Build history of the part. All positions in model axes, mm. Face numbers are marked on the shaded views. Round coordinates to 2 decimals unless told otherwise and drop trailing zeros. Write each loop counter-clockwise with the first axis right and the second up, starting at its lowest first coordinate (ties: lowest second). Pieces come first, ordered by that corner, then holes. Notation, with made-up numbers: M 41.25,43.5 L 49.25,43.5 A25 cw 49.25,65.5 Z; hole C 83,79 d2. An arc over 180 degrees is marked long. Use a Markdown table: item, result.
from build123d import *

# Parameters (mm, degrees)
SKETCH1_W           = 76.2
SKETCH1_H           = 50.8
SKETCH1_R           = 14.2748
BOSS_EXTRUDE1_DEPTH = 3.175
SKETCH2_R           = 22.225
BOSS_EXTRUDE2_DEPTH = 4.445
SKETCH3_R           = 14.2748
CUT_EXTRUDE1_DEPTH  = 92.688810795
SKETCH4_R           = 15.8623
CUT_EXTRUDE2_DEPTH  = 1.6002
FILLET1_R           = 2.54
FILLET2_R           = 2.54
SKETCH5_R           = 2.54
CUT_EXTRUDE3_DEPTH  = 92.688810795


with BuildPart() as part:
    # Sketch1 → Boss-Extrude1 (new body)
    with BuildSketch(Plane(origin=(0, 0, 0), x_dir=(1, 0, 0), z_dir=(0, 1, 0))):
        with Locations((38.1, 25.4)):
            Rectangle(SKETCH1_W, SKETCH1_H)
        with Locations(Location((38.1, 25.4, 0), (0, 0, 270))):
            Circle(SKETCH1_R, mode=Mode.SUBTRACT)
    extrude(amount=BOSS_EXTRUDE1_DEPTH)

    # Sketch2 → Boss-Extrude2 (add)
    with BuildSketch(Plane(origin=(0, 3.175, 0), x_dir=(1, 0, 0), z_dir=(0, 1, 0))):
        with Locations(Location((38.1, 25.4, 0), (0, 0, 90))):
            Circle(SKETCH2_R)
    extrude(amount=BOSS_EXTRUDE2_DEPTH)

    # Sketch3 → Cut-Extrude1 (cut, through all)
    with BuildSketch(Plane.XZ.offset(-3.175)):
        with Locations(Location((38.1, -25.4, 0), (0, 0, 270))):
            Circle(SKETCH3_R)
    extrude(amount=-CUT_EXTRUDE1_DEPTH, mode=Mode.SUBTRACT)

    # Sketch4 → Cut-Extrude2 (cut)
    with BuildSketch(Plane(origin=(0, 0, 0), x_dir=(-1, 0, 0), z_dir=(0, -1, 0))):
        with Locations(Location((-38.332507849, 25.4, 0), (0, 0, 90))):
            Circle(SKETCH4_R)
    extrude(amount=-CUT_EXTRUDE2_DEPTH, mode=Mode.SUBTRACT)

    # Fillet1
    fillet1_edges = [part.edges().sort_by_distance(p)[0] for p in [
        (38.1, 3.175, -3.175),
    ]]
    fillet(fillet1_edges, radius=FILLET1_R)

    # Fillet2
    fillet2_edges = [part.edges().sort_by_distance(p)[0] for p in [
        (0, 1.5875, -50.8),
        (76.2, 1.5875, -50.8),
        (76.2, 1.5875, 0),
        (0, 1.5875, 0),
    ]]
    fillet(fillet2_edges, radius=FILLET2_R)

    # Sketch5 → Cut-Extrude3 (cut, through all)
    with BuildSketch(Plane(origin=(0, 3.175, 0), x_dir=(1, 0, 0), z_dir=(0, 1, 0))):
        with Locations(Location((69.85, 41.275, 0), (0, 0, 270))):
            Circle(SKETCH5_R)
        with Locations(Location((69.85, 9.525, 0), (0, 0, 270))):
            Circle(SKETCH5_R)
        with Locations(Location((6.35, 9.525, 0), (0, 0, 270))):
            Circle(SKETCH5_R)
        with Locations(Location((6.35, 41.275, 0), (0, 0, 270))):
            Circle(SKETCH5_R)
    extrude(amount=-CUT_EXTRUDE3_DEPTH, mode=Mode.SUBTRACT)


solid = part.part
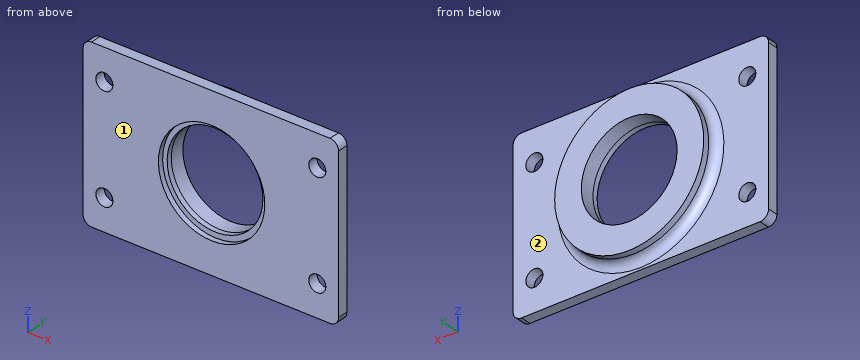
Q1. Drill centre lines: L1, parallel to X at y = 2.2, z = -25.4; L2, parallel to Y at x = 70, z = -20.5 (3 decimals); L3, parallel to Y at x = 27.5, z = -14. Where is each one in solid material? Low to high.
Response values:
| item | result |
|---|---|
| L1 | x = 0 to 23.83, 52.37 to 76.2 |
| L2 | y = 0 to 3.175 |
| L3 | y = 1.6 to 7.62 |
Q2. Cut at B-B on z = -25.4. Give the cut face in (x, y) (3 decimals), and give its area (3 significant figures).
Response values:
| item | result |
|---|---|
| outline | M 0,0 L 22.47,0 L 22.47,1.6 L 23.825,1.6 L 23.825,7.62 L 15.875,7.62 L 15.875,5.715 A2.54 cw 13.335,3.175 L 0,3.175 Z; M 52.375,1.6 L 54.195,1.6 L 54.195,0 L 76.2,0 L 76.2,3.175 L 62.865,3.175 A2.54 cw 60.325,5.715 L 60.325,7.62 L 52.375,7.62 Z |
| area | 220 mm2 |
Q3. Cut at A-A on x = 69.85. Give the cut face in (y, z) (3 decimals), and give its area (3 significant figures).
Response values:
| item | result |
|---|---|
| outline | M 0,-50.8 L 3.175,-50.8 L 3.175,-43.815 L 0,-43.815 Z; M 0,-38.735 L 3.175,-38.735 L 3.175,-12.065 L 0,-12.065 Z; M 0,-6.985 L 3.175,-6.985 L 3.175,0 L 0,0 Z |
| area | 129 mm2 |
Q4. Cut at C-C on x = 11.5. Give the cut face in (y, z) (3 decimals), and give its area (3 significant figures).
Response values:
| item | result |
|---|---|
| outline | M 0,-50.8 L 3.175,-50.8 L 3.175,0 L 0,0 Z |
| area | 161 mm2 |
Q5. Drop flat-ended pins along their axis: P1, Ø6, axis at x = 69.85, z = -41.275, coming from the +Y side (3 decimals); P2, Ø17, axis at x = 38.1, z = -25.4, coming from the -Y side; P3, Ø1, axis at y = 6, z = -9.5, coming from the +X side; P4, Ø2, axis at y = 5, z = -15, coming from the +X side. Give the stop position or say it passes through.
Response values:
| item | result |
|---|---|
| P1 | stops at y = 3.175 |
| P2 | passes through |
| P3 | stops at x = 54.12 |
| P4 | stops at x = 58.61 |
Q6. Two-plate mould, pull along Y, no slides. Class the marked faces 1 and 2: +Y half, -Y half, draft (parallel to the pull), parting line (faces both ways), or undercut.
Response values:
| item | result |
|---|---|
| face 1 | -Y half |
| face 2 | +Y half |
